```python
from build123d import *

# Parameters (mm, degrees)
SKETCH1_W                   = 70
SKETCH1_H                   = 30
BOSS_EXTRUDE1_DEPTH         = 56
CUT_EXTRUDE1_DEPTH          = 73.532751223
CUT_EXTRUDE2_DEPTH          = 68.720011813
CUT_EXTRUDE2_DEPTH_BACK     = 5
SKETCH3_R                   = 1.5
SKETCH4_R                   = 7.5
CUT_EXTRUDE5_DEPTH          = 10
SKETCH6_R                   = 15
CUT_EXTRUDE7_DEPTH          = 73.532751223
SKETCH7_W                   = 20
SKETCH7_H                   = 10
CUT_EXTRUDE8_DEPTH          = 10
CUT_EXTRUDE10_START         = -10
SKETCH8_R                   = 1.5
CUT_EXTRUDE10_DEPTH         = 10
CUT_EXTRUDE11_DEPTH         = 3
BOSS_EXTRUDE2_START         = -10
BOSS_EXTRUDE2_DEPTH         = 6
CHAMFER1_SIZE               = 0.5
CHAMFER2_SIZE               = 0.5
SKETCH10_W                  = 66
SKETCH10_H                  = 2
CUT_EXTRUDE13_DEPTH         = 3
CUT_EXTRUDE14_START         = -3
SKETCH12_W                  = 5
SKETCH12_H                  = 5
CUT_EXTRUDE14_DEPTH         = 3
BOSS_EXTRUDE3_START         = -24
BOSS_EXTRUDE3_DEPTH         = 24
TAP_DRILL_FOR_M3X0_5_TAP1_D = 2.5
FILLET1_R                   = 3


with BuildPart() as part:
    # Sketch1 → Boss-Extrude1 (new body)
    with BuildSketch(Plane(origin=(0, 0, 0), x_dir=(1, 0, 0), z_dir=(0, 1, 0))):
        Rectangle(SKETCH1_W, SKETCH1_H)
    extrude(amount=BOSS_EXTRUDE1_DEPTH)

    # Sketch2 → Cut-Extrude1 (cut, through all)
    with BuildSketch(Plane(origin=(0, 0, -15), x_dir=(-1, 0, 0), z_dir=(0, 0, -1))):
        with BuildLine():
            Line((32, 53), (-32, 53))
            Line((-32, 53), (-32, 45.748239349))
            ThreePointArc((-32, 45.748239349), (-17, 28), (-32, 10.251760651))
            Line((-32, 10.251760651), (-32, 3))
            Line((-32, 3), (32, 3))
            Line((32, 3), (32, 10.251760651))
            ThreePointArc((32, 10.251760651), (17, 28), (32, 45.748239349))
            Line((32, 45.748239349), (32, 53))
        make_face()
    extrude(amount=-CUT_EXTRUDE1_DEPTH, mode=Mode.SUBTRACT)

    # Sketch3 → Cut-Extrude2 (cut, two sides: drawn at the far end of the back side and taken through both)
    with BuildSketch(Plane.XZ.offset(-CUT_EXTRUDE2_DEPTH_BACK)):
        with Locations(Location((20, 0, 0), (0, 0, 90))):
            Circle(SKETCH3_R)
        with Locations(Location((-20, 0, 0), (0, 0, 90))):
            Circle(SKETCH3_R)
    extrude(amount=CUT_EXTRUDE2_DEPTH + CUT_EXTRUDE2_DEPTH_BACK, mode=Mode.SUBTRACT)

    # Sketch4 → Cut-Extrude5 (cut)
    with BuildSketch(Plane(origin=(35, 0, 0), x_dir=(0, 0, -1), z_dir=(1, 0, 0))):
        with Locations((0, 56)):
            Circle(SKETCH4_R)
        Circle(SKETCH4_R)
    cut_extrude5 = extrude(amount=-CUT_EXTRUDE5_DEPTH, mode=Mode.SUBTRACT)

    # Sketch6 → Cut-Extrude7 (cut, through all)
    with BuildSketch(Plane.XY.offset(15)):
        with Locations((-35, 28)):
            Circle(SKETCH6_R)
        with Locations((35, 28)):
            Circle(SKETCH6_R)
    extrude(amount=-CUT_EXTRUDE7_DEPTH, mode=Mode.SUBTRACT)

    # Sketch7 → Cut-Extrude8 (cut)
    with BuildSketch(Plane(origin=(0, 56, 0), x_dir=(1, 0, 0), z_dir=(0, 1, 0))):
        Rectangle(SKETCH7_W, SKETCH7_H)
    extrude(amount=-CUT_EXTRUDE8_DEPTH, mode=Mode.SUBTRACT)

    # Sketch8 → Cut-Extrude10 (cut)
    with BuildSketch(Plane(origin=(0, 56, 0), x_dir=(1, 0, 0), z_dir=(0, 1, 0)).offset(CUT_EXTRUDE10_START)):
        with Locations(Location((20, 0, 0), (0, 0, 270))):
            Circle(SKETCH8_R)
        with Locations(Location((-20, 0, 0), (0, 0, 270))):
            Circle(SKETCH8_R)
    extrude(amount=CUT_EXTRUDE10_DEPTH, mode=Mode.SUBTRACT)

    # Sketch2<3> → Cut-Extrude11 (cut)
    with BuildSketch(Plane(origin=(0, 0, -15), x_dir=(-1, 0, 0), z_dir=(0, 0, -1))):
        with BuildLine():
            Line((-33, 54), (-33, 44.881943016))
            ThreePointArc((-33, 44.881943016), (-18, 28), (-33, 11.118056984))
            Line((-33, 11.118056984), (-33, 2))
            Line((-33, 2), (33, 2))
            Line((33, 2), (33, 11.118056984))
            ThreePointArc((33, 11.118056984), (18, 28), (33, 44.881943016))
            Line((33, 44.881943016), (33, 54))
            Line((33, 54), (-33, 54))
        make_face()
        with BuildLine():
            Line((32, 53), (-32, 53))
            Line((-32, 53), (-32, 45.748239349))
            ThreePointArc((-32, 45.748239349), (-17, 28), (-32, 10.251760651))
            Line((-32, 10.251760651), (-32, 3))
            Line((-32, 3), (32, 3))
            Line((32, 3), (32, 10.251760651))
            ThreePointArc((32, 10.251760651), (17, 28), (32, 45.748239349))
            Line((32, 45.748239349), (32, 53))
        make_face(mode=Mode.SUBTRACT)
    cut_extrude11 = extrude(amount=-CUT_EXTRUDE11_DEPTH, mode=Mode.SUBTRACT)

    # Sketch11 → Boss-Extrude2 (add)
    with BuildSketch(Plane.XY.offset(15).offset(BOSS_EXTRUDE2_START)):
        with BuildLine():
            Line((-3, 3), (3, 3))
            Line((3, 3), (3, 25))
            Line((3, 25), (17.251760651, 25))
            ThreePointArc((17.251760651, 25), (17, 28), (17.251760651, 31))
            Line((17.251760651, 31), (3, 31))
            Line((3, 31), (3, 53))
            Line((3, 53), (-3, 53))
            Line((-3, 53), (-3, 31))
            Line((-3, 31), (-17.251760651, 31))
            ThreePointArc((-17.251760651, 31), (-17, 28), (-17.251760651, 25))
            Line((-17.251760651, 25), (-3, 25))
            Line((-3, 25), (-3, 3))
        make_face()
    extrude(amount=BOSS_EXTRUDE2_DEPTH)

    # Chamfer1
    chamfer1_edges = [part.edges().sort_by_distance(p)[0] for p in [
        (0, 56, 15),
        (32, 6.625880325, 15),
        (32, 49.374119675, 15),
        (0, 53, 15),
        (-32, 49.374119675, 15),
        (-17, 28, 15),
        (-32, 6.625880325, 15),
        (0, 3, 15),
        (17, 28, 15),
        (0, 0, 15),
        (35, 49.5, 15),
        (-35, 49.5, 15),
        (-35, 6.5, 15),
        (35, 6.5, 15),
        (-20, 28, 15),
        (20, 28, 15),
    ]]
    chamfer(chamfer1_edges, length=CHAMFER1_SIZE)

    # Chamfer2
    chamfer2_edges = [part.edges().sort_by_distance(p)[0] for p in [
        (0, 0, -15),
        (0, 56, -15),
        (-35, 49.5, -15),
        (35, 49.5, -15),
        (-35, 6.5, -15),
        (35, 6.5, -15),
        (-20, 28, -15),
        (20, 28, -15),
    ]]
    chamfer(chamfer2_edges, length=CHAMFER2_SIZE)

    # Sketch10 → Cut-Extrude13 (cut)
    with BuildSketch(Plane(origin=(0, 0, -15), x_dir=(-1, 0, 0), z_dir=(0, 0, -1))):
        with Locations((0, 55)):
            Rectangle(SKETCH10_W, SKETCH10_H)
    cut_extrude13 = extrude(amount=-CUT_EXTRUDE13_DEPTH, mode=Mode.SUBTRACT)

    # Mirror2: Cut-Extrude11, Cut-Extrude13 across plane
    add(cut_extrude11.mirror(Plane.XY), mode=Mode.SUBTRACT)
    add(cut_extrude13.mirror(Plane.XY), mode=Mode.SUBTRACT)

    # Sketch12 → Cut-Extrude14 (cut)
    with BuildSketch(Plane(origin=(35, 0, 0), x_dir=(0, 0, -1), z_dir=(1, 0, 0)).offset(CUT_EXTRUDE14_START)):
        with Locations((9.5, 7.5)):
            Rectangle(SKETCH12_W, SKETCH12_H)
        with Locations((9.5, 48.5)):
            Rectangle(SKETCH12_W, SKETCH12_H)
    cut_extrude14 = extrude(amount=CUT_EXTRUDE14_DEPTH, mode=Mode.SUBTRACT)

    # Mirror3: Cut-Extrude14 across plane
    add(cut_extrude14.mirror(Plane(origin=(0, 0, 0), x_dir=(0, 0, 1), z_dir=(1, 0, 0))), mode=Mode.SUBTRACT)

    # Mirror4: Cut-Extrude5 across plane
    add(cut_extrude5.mirror(Plane(origin=(0, 0, 0), x_dir=(0, 0, 1), z_dir=(1, 0, 0))), mode=Mode.SUBTRACT)

    # Sketch13 → Boss-Extrude3 (add)
    with BuildSketch(Plane(origin=(0, 0, -12), x_dir=(-1, 0, 0), z_dir=(0, 0, -1)).offset(BOSS_EXTRUDE3_START)):
        with BuildLine():
            Line((-2.236067977, 3), (2.236067977, 3))
            ThreePointArc((2.236067977, 3), (0, 8), (-2.236067977, 3))
        make_face()
        with BuildLine():
            ThreePointArc((-17.145915815, 30.287286146), (-12.204699164, 28), (-17.145915815, 25.712713854))
            ThreePointArc((-17.145915815, 25.712713854), (-17.001640796, 28), (-17.145915815, 30.287286146))
        make_face()
        with BuildLine():
            ThreePointArc((17.145915815, 30.287286146), (17.001640796, 28), (17.145915815, 25.712713854))
            ThreePointArc((17.145915815, 25.712713854), (12.204699164, 28), (17.145915815, 30.287286146))
        make_face()
    extrude(amount=BOSS_EXTRUDE3_DEPTH)

    # Tap Drill for M3x0.5 Tap1 (through all)
    with Locations(Plane(origin=(0, 0, -12), x_dir=(-1, 0, 0), z_dir=(0, 0, -1))):
        with Locations((-15.204699164, 28), (15.204699164, 28), (0, 5)):
            Hole(TAP_DRILL_FOR_M3X0_5_TAP1_D / 2)

    # Fillet1
    # the kernel refuses this fillet: 3 mm, written as the material it adds along each edge
    with BuildSketch(Plane(origin=(-17.145915815, 25.712713854, 12.276598744), x_dir=(-0.2068511279508174, -0.9783724295305314, 0), z_dir=(0, 0, -1))) as fillet1_piece_1_section:
        with BuildLine():
            CenterArc((3.153192789, -2.990178573), FILLET1_R, 94.637488492, 70.252161629)
            ThreePointArc((0.256916116, -2.208141853), (0.340537511, -1.079395596), (0, 0))
            ThreePointArc((0, 0), (1.455319749, -0.05892856), (2.910639498, 0))
        make_face()
    fillet1_piece_1 = extrude(amount=24.276598744, mode=Mode.PRIVATE)
    fillet1_piece_1 = split(fillet1_piece_1, bisect_by=Plane(origin=(-16.806719859, 24.740087729, 12), z_dir=(0, 0, -1)), keep=Keep.TOP, mode=Mode.PRIVATE)
    add(fillet1_piece_1)
    with BuildSketch(Plane(origin=(-17.145915815, 30.287286146, 12.276598744), x_dir=(-0.2068511279508151, 0.9783724295305319, 0), z_dir=(0, 0, -1))) as fillet1_piece_2_section:
        with BuildLine():
            CenterArc((3.153192789, 2.990178573), FILLET1_R, 195.110349879, 70.252161629)
            ThreePointArc((0.256916116, 2.208141853), (0.340537511, 1.079395596), (0, 0))
            ThreePointArc((0, 0), (1.455319749, 0.05892856), (2.910639498, 0))
        make_face()
    fillet1_piece_2 = extrude(amount=24.276598744, mode=Mode.PRIVATE)
    fillet1_piece_2 = split(fillet1_piece_2, bisect_by=Plane(origin=(-16.806719859, 31.259912271, 12), z_dir=(0, 0, -1)), keep=Keep.TOP, mode=Mode.PRIVATE)
    add(fillet1_piece_2)
    with BuildSketch(Plane(origin=(-2.236067977, 3, 14.200029514), x_dir=(-1, 0, 0), z_dir=(0, 0, -1))) as fillet1_piece_3_section:
        with BuildLine():
            CenterArc((3.680011806, 3), FILLET1_R, 189.594068227, 80.405931773)
            ThreePointArc((0.721971914, 2.5), (0.646151504, 1.167647394), (0, 0))
            Line((0, 0), (3.680011806, 0))
        make_face()
    fillet1_piece_3 = extrude(amount=26.200029514, mode=Mode.PRIVATE)
    fillet1_piece_3 = split(fillet1_piece_3, bisect_by=Plane(origin=(-3.476904083, 3.561012675, 12), z_dir=(0, 0, -1)), keep=Keep.TOP, mode=Mode.PRIVATE)
    add(fillet1_piece_3)
    with BuildSketch(Plane(origin=(2.236067977, 3, 14.200029514), x_dir=(1, 0, 0), z_dir=(0, 0, -1))) as fillet1_piece_4_section:
        with BuildLine():
            CenterArc((3.680011806, -3), FILLET1_R, 90, 80.405931773)
            ThreePointArc((0.721971914, -2.5), (0.646151504, -1.167647394), (0, 0))
            Line((0, 0), (3.680011806, 0))
        make_face()
    fillet1_piece_4 = extrude(amount=26.200029514, mode=Mode.PRIVATE)
    fillet1_piece_4 = split(fillet1_piece_4, bisect_by=Plane(origin=(3.476904083, 3.561012675, 12), z_dir=(0, 0, -1)), keep=Keep.TOP, mode=Mode.PRIVATE)
    add(fillet1_piece_4)
    with BuildSketch(Plane(origin=(17.145915815, 30.287286146, 12.276598744), x_dir=(0.20685112795081617, 0.9783724295305316, 0), z_dir=(0, 0, -1))) as fillet1_piece_5_section:
        with BuildLine():
            CenterArc((3.153192789, -2.990178573), FILLET1_R, 94.637488492, 70.252161629)
            ThreePointArc((0.256916116, -2.208141853), (0.340537511, -1.079395596), (0, 0))
            ThreePointArc((0, 0), (1.455319749, -0.05892856), (2.910639498, 0))
        make_face()
    fillet1_piece_5 = extrude(amount=24.276598744, mode=Mode.PRIVATE)
    fillet1_piece_5 = split(fillet1_piece_5, bisect_by=Plane(origin=(16.806719859, 31.259912271, 12), z_dir=(0, 0, -1)), keep=Keep.TOP, mode=Mode.PRIVATE)
    add(fillet1_piece_5)
    with BuildSketch(Plane(origin=(17.145915815, 25.712713854, 12.276598744), x_dir=(0.20685112795081684, -0.9783724295305316, 0), z_dir=(0, 0, -1))) as fillet1_piece_6_section:
        with BuildLine():
            CenterArc((3.153192789, 2.990178573), FILLET1_R, 195.110349879, 70.252161629)
            ThreePointArc((0.256916116, 2.208141853), (0.340537511, 1.079395596), (0, 0))
            ThreePointArc((0, 0), (1.455319749, 0.05892856), (2.910639498, 0))
        make_face()
    fillet1_piece_6 = extrude(amount=24.276598744, mode=Mode.PRIVATE)
    fillet1_piece_6 = split(fillet1_piece_6, bisect_by=Plane(origin=(16.806719859, 24.740087729, 12), z_dir=(0, 0, -1)), keep=Keep.TOP, mode=Mode.PRIVATE)
    add(fillet1_piece_6)


solid = part.part
```
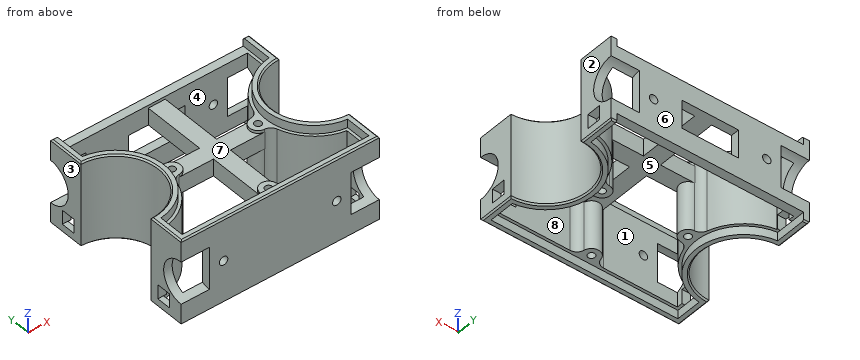
Work out the finished part from the listing and answer in its coordinate system (mm). Face numbers are marked on the shaded views. A direction names the side the tool comes from. Coordinates: 2 decimals unless noted, no trailing zeros. Use CSV: the item, a comma, the result in double quotes. Start each with the question number.
(1) Given pin 1 Ø5 at (y, z) = (27, 7.5) entering from +X; pin 2 Ø0.9 at (y, z) = (54, -3) entering from -X; pin 3 Ø1 at (x, y) = (-5, 35) entering from -Z; pin 4 Ø1 at (y, z) = (30.5, -1) entering from -X, each flat-ended and moving along its own axis, determine where each tip first touches the part or whether it passes through.
(2) For a pull along X with two mould halves and no side action, classify the marked faces 1, 2, 3 and 4 as +X half, -X half, draft (parallel to the pull), parting line (faces both ways), or undercut.
(3) For the marked faces 5, 6, 7 and 8, determine the directions among +Z, -Z, +X, -X, +Y, -Y from which every point of the face is accessible in a straight line to the end or side of a thin tool.
(4) Find section A-A, the plane y = 28. State how many separate pieces and enclosed holes the cut face has, then the cut area to 3 significant figures.
(5) Consider line 1 (X direction, y = 1.75, z = 0); line 2 (X direction, y = 54.3, z = 0); line 3 (Y direction, x = 8, z = -11.5). Determine where each line is inside the solid, lowest interval first.
Recorded:
1,pin 1,"stops at x = 20.41"
1,pin 2,"stops at x = -25"
1,pin 3,"passes through"
1,pin 4,"stops at x = -20.3"
2,face 1,"undercut"
2,face 2,"+X half"
2,face 3,"-X half"
2,face 4,"undercut"
3,face 5,"none"
3,face 6,"+Z, -Z, +X, -X, +Y"
3,face 7,"+Z"
3,face 8,"+Z, -Z"
4,separate pieces,"3"
4,enclosed holes,"0"
4,area,"424 mm^2"
5,line 1,"x = -25 to -21.5, -18.5 to 18.5, 21.5 to 25"
5,line 2,"x = -25 to -21.5, -18.5 to -10, 10 to 18.5, 21.5 to 25"
5,line 3,"y = 0 to 3, 53 to 56"
